Geometry: final body of the model. Coordinates: model frame, mm. Face numbers are marked on the shaded views. A direction names the side the tool comes from. Round coordinates to 2 decimals unless told otherwise and drop trailing zeros. Order: outer loops, then holes, each group sorted by start corner. A loop starts at its lowest first (then second) coordinate and runs counter-clockwise, first axis right, second up. Notation, with made-up numbers: (67, 60.25) - (111, 60.25) arc R10 cw to (111, 76.25) - close; hole circle Ø9 at (-35.5, 50). An arc over 180 degrees is marked (long way). Put each result on its own line as item: value. Start each with the question number.
(1) Pin query (flat end, axial travel): P1, Ø5, axis at x = 6.5, y = 38, coming from the -Z side; P2, Ø4.5, axis at y = 45.64, z = 40.5, coming from the +X side; P3, Ø8, axis at x = 42.5, z = 44, coming from the +Y side. Return the tip coordinate at first contact, or that it passes through.
(2) Pull-direction query (Z, two-part tool) for the marked faces 3, 4 and 5; classes: released by +Z, released by -Z, zero draft, split by the parting line, or undercut.
(3) Section B-B (x = 21). Output: boundary loops of the cut face in (y, z).
(4) Material intervals for L1, parallel to Z at x = 0.75, y = 45.5; L2, parallel to X at y = 3, z = 47, sorted ascending. Write a range as [from, to].
(5) Section A-A (z = 25). Output: boundary loops of the cut face in (x, y), and give its area (3 significant figures).
(6) Access query for the marked faces 1 and 2. Directions: +Z, -Z, +X, -X, +Y, -Y. A direction counts if a zero-diameter tool reaches every point of the face in a straight line with its end or side. Return the directions, or none.
(7) Section D-D (z = 40.5). Output: boundary loops of the cut face in (x, y), and give its area (3 significant figures).
(8) Section C-C (y = 30). Output: boundary loops of the cut face in (x, z), and give its area (3 significant figures).
from build123d import *

# Parameters (mm, degrees)
BOSS_EXTRUDE1_DEPTH = 50
SKETCH2_R           = 11.05
SKETCH2_R_2         = 2
CUT_EXTRUDE1_DEPTH  = 88.761039192
CUT_EXTRUDE2_DEPTH  = 50
BOSS_EXTRUDE2_DEPTH = 2
BOSS_EXTRUDE3_DEPTH = 2
CHAMFER1_SIZE       = 5
SKETCH8_R           = 1.3611534
CUT_EXTRUDE3_DEPTH  = 10


with BuildPart() as part:
    # Sketch1 → Boss-Extrude1 (new body)
    with BuildSketch(Plane.XY):
        Polygon((0, 0), (0, 51), (2, 51), (2, 2), (53, 2), (53, 0), align=None)
    extrude(amount=BOSS_EXTRUDE1_DEPTH)

    # Sketch2 → Cut-Extrude1 (cut, through all)
    with BuildSketch(Plane(origin=(2, 0, 0), x_dir=(0, 0, -1), z_dir=(1, 0, 0))):
        with Locations(Location((-25, 30, 0), (0, 0, 90))):
            Circle(SKETCH2_R)
        with Locations(Location((-40.5, 45.640445987, 0), (0, 0, 90))):
            Circle(SKETCH2_R_2)
        with Locations(Location((-9.5, 45.5, 0), (0, 0, 90))):
            Circle(SKETCH2_R_2)
        with Locations(Location((-40.5, 14.5, 0), (0, 0, 90))):
            Circle(SKETCH2_R_2)
        with Locations(Location((-9.5, 14.5, 0), (0, 0, 90))):
            Circle(SKETCH2_R_2)
    extrude(amount=-CUT_EXTRUDE1_DEPTH, mode=Mode.SUBTRACT)

    # Sketch3 → Cut-Extrude2 (cut)
    with BuildSketch(Plane(origin=(0, 2, 0), x_dir=(1, 0, 0), z_dir=(0, 1, 0))):
        with BuildLine():
            Line((12.455251015, -12.1), (42.544748985, -12.1))
            ThreePointArc((42.544748985, -12.1), (44.644629774, -9.977624237), (42.5, -7.900476833))
            Line((42.5, -7.900476833), (12.5, -7.900476833))
            ThreePointArc((12.5, -7.900476833), (10.355370226, -9.977624237), (12.455251015, -12.1))
        make_face()
        with BuildLine():
            Line((12.5, -42.099523167), (42.5, -42.099523167))
            ThreePointArc((42.5, -42.099523167), (44.644629774, -40.022375763), (42.544748985, -37.9))
            Line((42.544748985, -37.9), (12.455251015, -37.9))
            ThreePointArc((12.455251015, -37.9), (10.355370226, -40.022375763), (12.5, -42.099523167))
        make_face()
    extrude(amount=-CUT_EXTRUDE2_DEPTH, mode=Mode.SUBTRACT)

    # Sketch5 → Boss-Extrude2 (add)
    with BuildSketch(Plane.XY.offset(50)):
        Polygon((2, 22), (2, 4), (4, 2), (15, 2), align=None)
    extrude(amount=-BOSS_EXTRUDE2_DEPTH)

    # Sketch6 → Boss-Extrude3 (add)
    with BuildSketch(Plane(origin=(0, 0, 0), x_dir=(-1, 0, 0), z_dir=(0, 0, -1))):
        Polygon((-4, 2), (-2, 4), (-2, 22), (-15, 2), align=None)
    extrude(amount=-BOSS_EXTRUDE3_DEPTH)

    # Chamfer1
    chamfer1_edges = [part.edges().sort_by_distance(p)[0] for p in [
        (1, 51, 50),
        (1, 51, 0),
        (53, 1, 50),
        (53, 1, 0),
    ]]
    chamfer(chamfer1_edges, length=CHAMFER1_SIZE)

    # Sketch8 → Cut-Extrude3 (cut)
    with BuildSketch(Plane.ZY):
        with Locations(Location((35.606601718, 19.393398282, 0), (0, 0, 270))):
            Circle(SKETCH8_R)
        with Locations(Location((14.393398282, 19.393398282, 0), (0, 0, 270))):
            Circle(SKETCH8_R)
        with Locations(Location((14.393398282, 40.606601718, 0), (0, 0, 270))):
            Circle(SKETCH8_R)
        with Locations(Location((35.606601718, 40.606601718, 0), (0, 0, 270))):
            Circle(SKETCH8_R)
    extrude(amount=-CUT_EXTRUDE3_DEPTH, mode=Mode.SUBTRACT)


solid = part.part
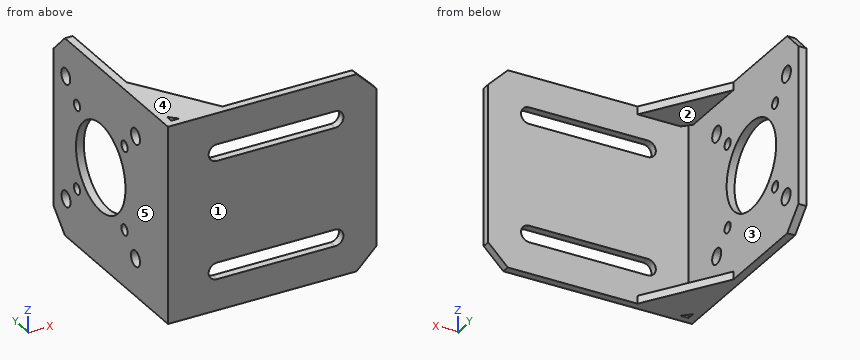
Checks:
1. P1: passes through
1. P2: stops at x = 2
1. P3: stops at y = 2
2. face 3: undercut
2. face 4: released by +Z
2. face 5: zero draft
3. outline: (0, 0) - (2, 0) - (2, 7.9) - (0, 7.9) - close; (0, 12.1) - (2, 12.1) - (2, 37.9) - (0, 37.9) - close; (0, 42.1) - (2, 42.1) - (2, 50) - (0, 50) - close
4. L1: z = [0, 7.5], [11.5, 38.5], [42.5, 50]
4. L2: x = [0, 2]
5. outline: (0, 0) - (53, 0) - (53, 2) - (2, 2) - (2, 18.95) - (0, 18.95) - close; (0, 41.05) - (2, 41.05) - (2, 51) - (0, 51) - close
5. area: 160 mm²
6. face 1: +Z, -Z, +X, -X, -Y
6. face 2: +X, +Y
7. outline: (0, 0) - (10.42, 0) - (10.42, 2) - (2, 2) - (2, 12.5) - (0, 12.5) - close; (0, 16.5) - (2, 16.5) - (2, 43.64) - (0, 43.64) - close; (0, 47.64) - (2, 47.64) - (2, 51) - (0, 51) - close; (44.58, 0) - (53, 0) - (53, 2) - (44.58, 2) - close
7. area: 120 mm²
8. outline: (0, 0) - (2, 0) - (2, 13.95) - (0, 13.95) - close; (0, 36.05) - (2, 36.05) - (2, 50) - (0, 50) - close
8. area: 55.8 mm²
